Part model, mm, in its own coordinate system. Face numbers are marked on the shaded views. A direction names the side the tool comes from. Round coordinates to 2 decimals unless told otherwise and drop trailing zeros. Write each loop counter-clockwise with the first axis right and the second up, starting at its lowest first coordinate (ties: lowest second). Pieces come first, ordered by that corner, then holes. Notation, with made-up numbers: (27, -21.75) -> (66, -21.75) arc R16 cw to (66, -11.75) -> close; hole circle Ø7 at (68.25, 19.25). An arc over 180 degrees is marked (long way). Return JSON: item names as keys, results as strings. Group by question number.
```python
from build123d import *

# Parameters (mm, degrees)
SKETCH1_W           = 246
SKETCH1_H           = 154
BOSS_EXTRUDE1_DEPTH = 7
SKETCH2_W           = 240
SKETCH2_H           = 148
CUT_EXTRUDE1_DEPTH  = 5
SKETCH3_W           = 220
SKETCH3_H           = 128
CUT_EXTRUDE2_DEPTH  = 5
BOSS_EXTRUDE2_START = -3
SKETCH6_W           = 246
SKETCH6_H           = 154
BOSS_EXTRUDE2_DEPTH = 2.5
SKETCH8_W           = 39
SKETCH8_H           = 0.3
SKETCH8_W_2         = 12.26
CUT_EXTRUDE5_DEPTH  = 5
SKETCH9_R           = 0.5
CUT_EXTRUDE6_DEPTH  = 5
SKETCH10_R          = 2.54
CUT_EXTRUDE7_DEPTH  = 5
SKETCH11_W          = 249.3
SKETCH11_H          = 253.3
SKETCH11_W_2        = 245.3
SKETCH11_H_2        = 249.3
BOSS_EXTRUDE3_DEPTH = 22
BOSS_EXTRUDE3_DRAFT = -2
SKETCH12_R          = 1.7
CUT_EXTRUDE8_DEPTH  = 332.406096652
SKETCH13_R          = 1.7
CUT_EXTRUDE9_DEPTH  = 310.160818194
SKETCH14_W          = 120
SKETCH14_H          = 50
BOSS_EXTRUDE4_DEPTH = 15
CUT_EXTRUDE10_START = -2
SKETCH15_W          = 116
SKETCH15_H          = 46
CUT_EXTRUDE10_DEPTH = 239.282125844
FILLET1_R           = 2
CUT_EXTRUDE11_DEPTH = 241.656394056


with BuildPart() as part:
    # Sketch1 → Boss-Extrude1 (new body)
    with BuildSketch(Plane(origin=(0, 0, 0), x_dir=(1, 0, 0), z_dir=(0, 1, 0))):
        Rectangle(SKETCH1_W, SKETCH1_H)
    extrude(amount=-BOSS_EXTRUDE1_DEPTH)

    # Sketch2 → Cut-Extrude1 (cut)
    with BuildSketch(Plane(origin=(0, 0, 0), x_dir=(1, 0, 0), z_dir=(0, 1, 0))):
        Rectangle(SKETCH2_W, SKETCH2_H)
    extrude(amount=-CUT_EXTRUDE1_DEPTH, mode=Mode.SUBTRACT)

    # Sketch3 → Cut-Extrude2 (cut)
    with BuildSketch(Plane(origin=(0, -5, 0), x_dir=(1, 0, 0), z_dir=(0, 1, 0))):
        Rectangle(SKETCH3_W, SKETCH3_H)
    extrude(amount=-CUT_EXTRUDE2_DEPTH, mode=Mode.SUBTRACT)

    # Sketch6 → Boss-Extrude2 (add)
    with BuildSketch(Plane(origin=(0, 0, 0), x_dir=(1, 0, 0), z_dir=(0, 1, 0)).offset(BOSS_EXTRUDE2_START)):
        with BuildLine():
            Line((-128.49, -99.5), (128.49, -99.5))
            ThreePointArc((128.49, -99.5), (140.164332957, -94.664332957), (145, -82.99))
            Line((145, -82.99), (145, 173.99))
            ThreePointArc((145, 173.99), (140.164332957, 185.664332957), (128.49, 190.5))
            Line((128.49, 190.5), (-128.49, 190.5))
            ThreePointArc((-128.49, 190.5), (-140.164332957, 185.664332957), (-145, 173.99))
            Line((-145, 173.99), (-145, -82.99))
            ThreePointArc((-145, -82.99), (-140.164332957, -94.664332957), (-128.49, -99.5))
        make_face()
        Rectangle(SKETCH6_W, SKETCH6_H, mode=Mode.SUBTRACT)
    extrude(amount=-BOSS_EXTRUDE2_DEPTH)

    # Sketch8 → Cut-Extrude5 (cut)
    with BuildSketch(Plane(origin=(0, -5, 0), x_dir=(1, 0, 0), z_dir=(0, 1, 0))):
        with Locations((0.5, -72.95)):
            Rectangle(SKETCH8_W, SKETCH8_H)
        with Locations((-36.13, -72.95)):
            Rectangle(SKETCH8_W_2, SKETCH8_H)
    extrude(amount=-CUT_EXTRUDE5_DEPTH, mode=Mode.SUBTRACT)

    # Sketch9 → Cut-Extrude6 (cut)
    with BuildSketch(Plane(origin=(0, -5, 0), x_dir=(1, 0, 0), z_dir=(0, 1, 0))):
        with Locations(Location((119, -46.2, 0), (0, 0, 270))):
            Circle(SKETCH9_R)
        with Locations(Location((119, -42.7, 0), (0, 0, 270))):
            Circle(SKETCH9_R)
    extrude(amount=-CUT_EXTRUDE6_DEPTH, mode=Mode.SUBTRACT)

    # Sketch10 → Cut-Extrude7 (cut)
    with BuildSketch(Plane(origin=(0, -3, 0), x_dir=(1, 0, 0), z_dir=(0, 1, 0))):
        with Locations(Location((-133.604, 140.242, 0), (0, 0, 270))):
            Circle(SKETCH10_R)
        with Locations(Location((-106.172, 180.12, 0), (0, 0, 270))):
            Circle(SKETCH10_R)
        with Locations(Location((-133.604, -49.242, 0), (0, 0, 90))):
            Circle(SKETCH10_R)
        with Locations(Location((-133.604, 45.5, 0), (0, 0, 270))):
            Circle(SKETCH10_R)
        with Locations(Location((0, 180.12, 0), (0, 0, 270))):
            Circle(SKETCH10_R)
        with Locations(Location((0, -89.12, 0), (0, 0, 90))):
            Circle(SKETCH10_R)
        with Locations(Location((-106.172, -89.12, 0), (0, 0, 90))):
            Circle(SKETCH10_R)
        with Locations(Location((106.172, -89.12, 0), (0, 0, 270))):
            Circle(SKETCH10_R)
        with Locations(Location((133.604, 45.5, 0), (0, 0, 90))):
            Circle(SKETCH10_R)
        with Locations(Location((133.604, -49.242, 0), (0, 0, 270))):
            Circle(SKETCH10_R)
        with Locations(Location((106.172, 180.12, 0), (0, 0, 90))):
            Circle(SKETCH10_R)
        with Locations(Location((133.604, 140.242, 0), (0, 0, 90))):
            Circle(SKETCH10_R)
    extrude(amount=-CUT_EXTRUDE7_DEPTH, mode=Mode.SUBTRACT)


with BuildPart() as boss_extrude3_tool:
    # Sketch11 → Boss-Extrude3 (with draft: the straight prism first)
    with BuildSketch(Plane.XZ.offset(5.5)):
        with Locations((0, -45.5)):
            Rectangle(SKETCH11_W, SKETCH11_H)
        with Locations((0, -45.5)):
            Rectangle(SKETCH11_W_2, SKETCH11_H_2, mode=Mode.SUBTRACT)
    extrude(amount=BOSS_EXTRUDE3_DEPTH)
    # Boss-Extrude3: the draft: its side faces are tilted about the plane it starts from
    boss_extrude3_sides = [boss_extrude3_tool.faces().sort_by_distance(p)[0] for p in [
        (0, -16.5, -172.15),
        (124.65, -16.5, -45.5),
        (0, -16.5, 81.15),
        (-124.65, -16.5, -45.5),
        (0, -16.5, 79.15),
        (122.65, -16.5, -45.5),
        (0, -16.5, -170.15),
        (-122.65, -16.5, -45.5),
    ]]
    draft(boss_extrude3_sides, Plane.XZ.offset(5.5), BOSS_EXTRUDE3_DRAFT)


with BuildPart() as part_1:
    add(part.part)

    # Boss-Extrude3: add boss_extrude3_tool
    add(boss_extrude3_tool.part)

    # Sketch12 → Cut-Extrude8 (cut, through all)
    with BuildSketch(Plane(origin=(124.30634913, 4.340873364, 0), x_dir=(0, 0, -1), z_dir=(0.9993908270190958, 0.03489949670250105, 0))):
        with Locations(Location((-49.5, -16.860281787, 0), (0, 0, 90))):
            Circle(SKETCH12_R)
        with Locations(Location((140.5, -16.860281787, 0), (0, 0, 90))):
            Circle(SKETCH12_R)
    extrude(amount=-CUT_EXTRUDE8_DEPTH, mode=Mode.SUBTRACT)

    # Sketch13 → Cut-Extrude9 (cut, through all)
    with BuildSketch(Plane(origin=(0, 2.82367006, 80.859331036), x_dir=(1, 0, 0), z_dir=(0, 0.03489949670250106, 0.9993908270190958))):
        with Locations(Location((-95, -15.342153681, 0), (0, 0, 270))):
            Circle(SKETCH13_R)
        with Locations(Location((95, -15.342153681, 0), (0, 0, 90))):
            Circle(SKETCH13_R)
    extrude(amount=-CUT_EXTRUDE9_DEPTH, mode=Mode.SUBTRACT)

    # Sketch14 → Boss-Extrude4 (add)
    with BuildSketch(Plane.XZ.offset(5.5)):
        with Locations((50, -133.75)):
            Rectangle(SKETCH14_W, SKETCH14_H)
    extrude(amount=BOSS_EXTRUDE4_DEPTH)

    # Sketch15 → Cut-Extrude10 (cut, through all)
    with BuildSketch(Plane.XZ.offset(20.5).offset(CUT_EXTRUDE10_START)):
        with Locations((50, -133.75)):
            Rectangle(SKETCH15_W, SKETCH15_H)
    extrude(amount=-CUT_EXTRUDE10_DEPTH, mode=Mode.SUBTRACT)

    # Fillet1
    fillet1_edges = [part_1.edges().sort_by_distance(p)[0] for p in [
        (108, -18.5, -133.75),
        (50, -18.5, -110.75),
        (-8, -18.5, -133.75),
        (50, -18.5, -156.75),
    ]]
    fillet(fillet1_edges, radius=FILLET1_R)

    # Sketch16 → Cut-Extrude11 (cut, through all)
    with BuildSketch(Plane(origin=(0, -3, 0), x_dir=(1, 0, 0), z_dir=(0, 1, 0))):
        Polygon((-57.298294078, 150.5), (-63.649147039, 161.5), (-76.350852961, 161.5), (-82.701705922, 150.5), (-76.350852961, 139.5), (-63.649147039, 139.5), align=None)
        Polygon((-84.030344885, 117), (-89.515172443, 126.5), (-100.484827557, 126.5), (-105.969655115, 117), (-100.484827557, 107.5), (-89.515172443, 107.5), align=None)
        with BuildLine():
            Line((-51.23, 119.85), (-38.77, 119.85))
            ThreePointArc((-38.77, 119.85), (-38.550796898, 119.759203102), (-38.46, 119.54))
            Line((-38.46, 119.54), (-38.46, 114.46))
            ThreePointArc((-38.46, 114.46), (-38.550796898, 114.240796898), (-38.77, 114.15))
            Line((-38.77, 114.15), (-51.23, 114.15))
            ThreePointArc((-51.23, 114.15), (-51.449203102, 114.240796898), (-51.54, 114.46))
            Line((-51.54, 114.46), (-51.54, 119.54))
            ThreePointArc((-51.54, 119.54), (-51.449203102, 119.759203102), (-51.23, 119.85))
        make_face()
    extrude(amount=-CUT_EXTRUDE11_DEPTH, mode=Mode.SUBTRACT)


solid = part_1.part
```
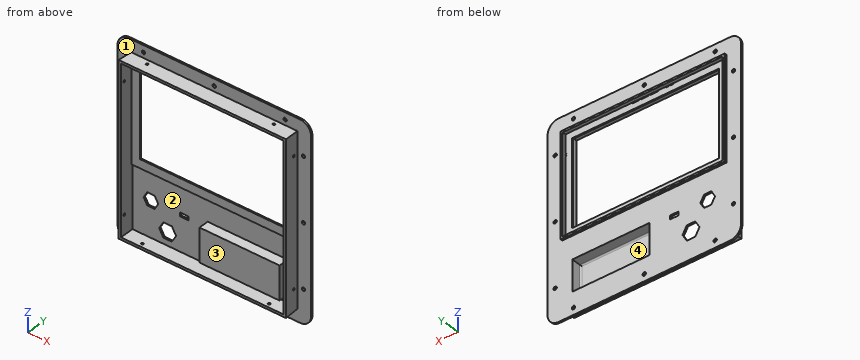
Item 1: Flat gauge pins, fed straight in: P1, Ø4, axis at x = 106, y = -21, coming from the -Z side; P2, Ø3, axis at x = -78, y = -21, coming from the -Z side; P3, Ø2, axis at y = -16.5, z = 11, coming from the +X side; P4, Ø1.6, axis at x = -6.5, y = -6, coming from the -Z side. Where does each tip first touch, or does it go through?
Item 2: Two-plate mould, pull along Z, no slides. Class the marked faces 1 and 2: released by +Z, released by -Z, zero draft, split by the parting line, or undercut.
Item 3: Which spindle directions (+Z, -Z, +X, -X, +Y, -Y) get a long thin tool onto all of the face, cutting with end or side? Do the marked faces 3 and 4. Say none if no direction does.
Item 4: Cut at A-A (z = -26). Write the cut outline in (x, y).
Item 5: Wall check: L1, parallel to Z at x = 96, y = -3.5; L2, parallel to Z at x = 119, y = -6.15; L3, parallel to X at y = -3.7, z = -45.5. Give the ranges that are in metal, low to high.
Checks:
{
 "1": {"P1": "stops at z = -172.76", "P2": "stops at z = -172.74", "P3": "stops at x = 125.07", "P4": "stops at z = -190.5"},
 "2": {"face 1": "zero draft", "face 2": "undercut"},
 "3": {"face 3": "-Y", "face 4": "+Y"},
 "4": {"outline": "(-145, -5.5) -> (-124.65, -5.5) -> (-125.42, -27.5) -> (-121.88, -27.5) -> (-122.6, -7) -> (-110, -7) -> (-110, -5) -> (-120, -5) -> (-120, 0) -> (-123, 0) -> (-123, -3) -> (-145, -3) -> close; (110, -7) -> (122.6, -7) -> (121.88, -27.5) -> (125.42, -27.5) -> (124.65, -5.5) -> (145, -5.5) -> (145, -3) -> (123, -3) -> (123, 0) -> (120, 0) -> (120, -5) -> (110, -5) -> close"},
 "5": {"L1": "z = -190.5 to -156.75, -110.75 to -74, 74 to 99.5", "L2": "z = -172.17 to -170.13, -77 to 42.2, 43.2 to 45.7, 46.7 to 77, 79.13 to 81.17", "L3": "x = -145 to -136.14, -131.06 to -120, 120 to 131.06, 136.14 to 145"}
}
